Build history of the part. All positions in model axes, mm. Face numbers are marked on the shaded views. A direction names the side the tool comes from. Give positions to 0.01 mm unless a question says otherwise; leave off trailing zeros. Loops run counter-clockwise (first coordinate to the right, second up) from the corner with the lowest first, then second, coordinate; pieces in that order, holes last. Notation, with made-up numbers: (79, 32.5) -> (115, 32.5) arc R21 ccw to (115, 67.5) -> close; hole circle Ø1 at (-27.75, 19.25). An arc over 180 degrees is marked (long way). One line per question, with ' | ' between items. Start each with the question number.
(1) Slice it at A-A, the plane y = -26. Write the cut outline in (x, z).
(2) Drill centre lines: L1, parallel to Y at x = 23, z = 0; L2, parallel to Y at x = 16, z = 0; L3, parallel to Y at x = 27, z = 14. Where is each one in solid material? Low to high. Write a range as from..to.
(3) Slice it at B-B, the plane y = -6. Write the cut outline in (x, z), then the cut area to 3 significant figures.
(4) Mould opens along Z. For the marked faces 1, 2 and 3 say: pulls with the +Z half, pulls with the -Z half, needs draft (parallel to the pull), parting line crosses it, or undercut.
(5) Slice it at D-D, the plane z = 0. Give the number of separate pieces and of enclosed holes in the cut face, then the cut area to 3 significant figures.
(6) Flat gauge pins, fed straight in: pin 1 Ø8 at (y, z) = (-10, 10) entering from +X; pin 2 Ø6.5 at (x, y) = (4.5, -4) entering from -Z; pin 3 Ø4 at (y, z) = (-18.5, 5.5) entering from -X; pin 4 Ø6 at (y, z) = (-8.25, 0) entering from -X. Where does each tip first touch, or does it go through?
(7) 3-axis set-ups, long thin cutter, end or side, ignore diameter. For the marked faces 4, 5, 6, 7 and 8: which of +Z, -Z, +X, -X, +Y, -Y reach the whole face in a straight line?
(8) Slice it at C-C, the plane y = -32. Write the cut outline in (x, z), then the cut area to 3 significant figures.
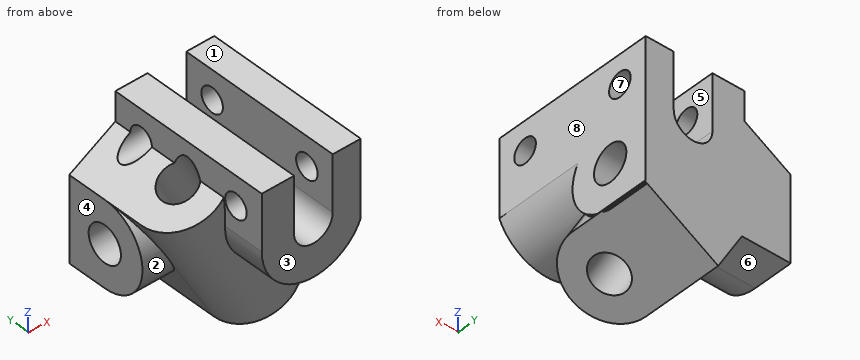
```python
from build123d import *

# Parameters (mm, degrees)
SKETCH1_R               = 3.75
BOSS_EXTRUDE1_DEPTH     = 30
SKETCH2_R               = 3.75
BOSS_EXTRUDE2_DEPTH     = 30
CUT_EXTRUDE1_DEPTH      = 26.5000001
SKETCH4_W               = 5.792740578
SKETCH4_H               = 11.5
BOSS_EXTRUDE3_DEPTH     = 10
BOSS_EXTRUDE4_DEPTH     = 10
BOSS_EXTRUDE5_DEPTH     = 34
SKETCH5_R               = 2.5
CUT_EXTRUDE2_DEPTH      = 31.0000001
SKETCH7_R               = 3.75
CUT_EXTRUDE3_DEPTH      = 31.155444666
SKETCH8_R               = 3.75
CUT_EXTRUDE4_DEPTH      = 27.5
CUT_EXTRUDE4_DEPTH_BACK = 38.57772242


with BuildPart() as part:
    # Sketch1 → Boss-Extrude1 (new body)
    with BuildSketch(Plane(origin=(0, 0, 0), x_dir=(0, 0, -1), z_dir=(1, 0, 0))):
        with BuildLine():
            Line((-8.75, 0), (8.75, 0))
            Line((8.75, 0), (8.75, 8.25))
            ThreePointArc((8.75, 8.25), (0, 17), (-8.75, 8.25))
            Line((-8.75, 8.25), (-8.75, 0))
        make_face()
        with Locations((0, 8.25)):
            Circle(SKETCH1_R, mode=Mode.SUBTRACT)
    extrude(amount=BOSS_EXTRUDE1_DEPTH)

    # Sketch2 → Boss-Extrude2 (add)
    with BuildSketch(Plane(origin=(-3.788861142, 0, 6.5625), x_dir=(-0.866025404, 0, -0.5), z_dir=(0.5, 0, -0.866025404))):
        with BuildLine():
            Line((-4.375, 0), (-4.375, 16.75))
            ThreePointArc((-4.375, 16.75), (-13.125, 25.5), (-21.875, 16.75))
            Line((-21.875, 16.75), (-21.875, 0))
            Line((-21.875, 0), (-4.375, 0))
        make_face()
        with Locations((-13.125, 16.75)):
            Circle(SKETCH2_R, mode=Mode.SUBTRACT)
    extrude(amount=BOSS_EXTRUDE2_DEPTH)

    # Sketch3 → Cut-Extrude1 (cut, through all)
    with BuildSketch(Plane.XZ):
        with BuildLine():
            Line((24.207259422, 8.75), (24.207259422, 15.67820323))
            Line((24.207259422, 15.67820323), (16.207259422, 15.67820323))
            Line((16.207259422, 15.67820323), (16.207259422, 8.75))
            ThreePointArc((16.207259422, 8.75), (20.207259422, 4.75), (24.207259422, 8.75))
        make_face()
    extrude(amount=-CUT_EXTRUDE1_DEPTH, mode=Mode.SUBTRACT)

    # Sketch4 → Boss-Extrude3 (add)
    with BuildSketch(Plane.XZ):
        with Locations((27.103629711, 14.5)):
            Rectangle(SKETCH4_W, SKETCH4_H)
    extrude(amount=-BOSS_EXTRUDE3_DEPTH)

    # Sketch6 → Boss-Extrude4 (add)
    with BuildSketch(Plane.XZ):
        Polygon((16.207259422, 15.67820323), (16.207259422, 20.25), (9.526279442, 20.25), (9.526279442, 14.25), align=None)
    extrude(amount=-BOSS_EXTRUDE4_DEPTH)

    # Sketch9 → Boss-Extrude5 (add)
    with BuildSketch(Plane.XZ):
        with BuildLine():
            Line((16.207259422, 20.25), (9.526279442, 20.25))
            Line((9.526279442, 20.25), (9.526279442, 14.25))
            Line((9.526279442, 14.25), (9.526279442, 8.75))
            ThreePointArc((9.526279442, 8.75), (18.029270984, -1.706562518), (30, 4.485546307))
            Line((30, 4.485546307), (30, 20.25))
            Line((30, 20.25), (24.207259422, 20.25))
            Line((24.207259422, 20.25), (24.207259422, 8.75))
            ThreePointArc((24.207259422, 8.75), (20.207259422, 4.75), (16.207259422, 8.75))
            Line((16.207259422, 8.75), (16.207259422, 20.25))
        make_face()
    extrude(amount=-BOSS_EXTRUDE5_DEPTH)

    # Sketch5 → Cut-Extrude2 (cut, through all)
    with BuildSketch(Plane(origin=(30, 0, 0), x_dir=(0, 0, -1), z_dir=(1, 0, 0))):
        with Locations(Location((-14.25, 6, 0), (0, 0, 90))):  # turned: the seam where the file's is
            Circle(SKETCH5_R)
        with Locations(Location((-14.25, 28, 0), (0, 0, 180))):  # turned: the seam where the file's is
            Circle(SKETCH5_R)
    extrude(amount=-CUT_EXTRUDE2_DEPTH, mode=Mode.SUBTRACT)

    # Sketch7 → Cut-Extrude3 (cut, through all)
    with BuildSketch(Plane.ZY):
        with Locations(Location((0, 8.25, 0), (0, 0, 180))):  # turned: the seam where the file's is
            Circle(SKETCH7_R)
    extrude(amount=-CUT_EXTRUDE3_DEPTH, mode=Mode.SUBTRACT)

    # Sketch8 → Cut-Extrude4 (cut, two sides)
    with BuildSketch(Plane(origin=(-3.788861142, 0, 6.5625), x_dir=(0.866025404, 0, 0.5), z_dir=(-0.5, 0, 0.866025404))) as cut_extrude4_sk:
        with Locations(Location((13.125, 16.75, 0), (0, 0, 53.130102354))):  # turned: the seam where the file's is
            Circle(SKETCH8_R)
    extrude(amount=CUT_EXTRUDE4_DEPTH, mode=Mode.SUBTRACT)
    extrude(cut_extrude4_sk.sketch, amount=-CUT_EXTRUDE4_DEPTH_BACK, mode=Mode.SUBTRACT)


with BuildPart() as body_2:
    # Mirror1: mirrored copy
    add(part.part.mirror(Plane(origin=(30, 0, 8.75), x_dir=(0, 0, 1), z_dir=(0, 1, 0))))


solid = body_2.part
```
Final values:
1) outline: (9.53, 8.75) arc R10.68 ccw to (30, 4.49) -> (30, 12.75) -> (24.21, 12.75) -> (24.21, 8.75) arc R4 cw to (16.21, 8.75) -> (16.21, 12.75) -> (9.53, 12.75) -> close; (9.53, 15.75) -> (16.21, 15.75) -> (16.21, 20.25) -> (9.53, 20.25) -> close; (24.21, 15.75) -> (30, 15.75) -> (30, 20.25) -> (24.21, 20.25) -> close
2) L1: -34..-12, -4.5..0 | L2: -34..-20.43, -13.07..-12, -4.5..0 | L3: -34..-30.49, -25.51..-8.49, -3.51..0
3) outline: (0, -8.75) -> (10.1, -8.75) -> (15, -17.23) -> (29.69, -8.75) -> (30, -8.75) -> (30, -8.57) -> (30.16, -8.48) -> (30, -8.21) -> (30, -3) -> (0, -3) -> close; (0, 3) -> (30, 3) -> (30, 11.75) -> (24.21, 11.75) -> (24.21, 8.75) arc R4 cw to (16.21, 8.75) -> (16.21, 11.75) -> (5.2, 11.75) -> (0, 8.75) -> close; (9.53, 16.75) -> (16.21, 16.75) -> (16.21, 20.25) -> (9.53, 20.25) -> close; (24.21, 16.75) -> (30, 16.75) -> (30, 20.25) -> (24.21, 20.25) -> close | area: 505 mm2
4) face 1: pulls with the +Z half | face 2: undercut | face 3: needs draft
5) separate pieces: 2 | enclosed holes: 1 | area: 500 mm2
6) pin 1: x = 30 | pin 2: z = -8.75 | pin 3: x = 0.86 | pin 4: through
7) face 4: +Z, -Z, -X, +Y, -Y | face 5: +Z, +Y, -Y | face 6: -Z, -X, +Y, -Y | face 7: +X, -X | face 8: +Z, +X, +Y, -Y
8) outline: (9.53, 8.75) arc R10.68 ccw to (30, 4.49) -> (30, 20.25) -> (24.21, 20.25) -> (24.21, 8.75) arc R4 cw to (16.21, 8.75) -> (16.21, 20.25) -> (9.53, 20.25) -> close | area: 295 mm2
